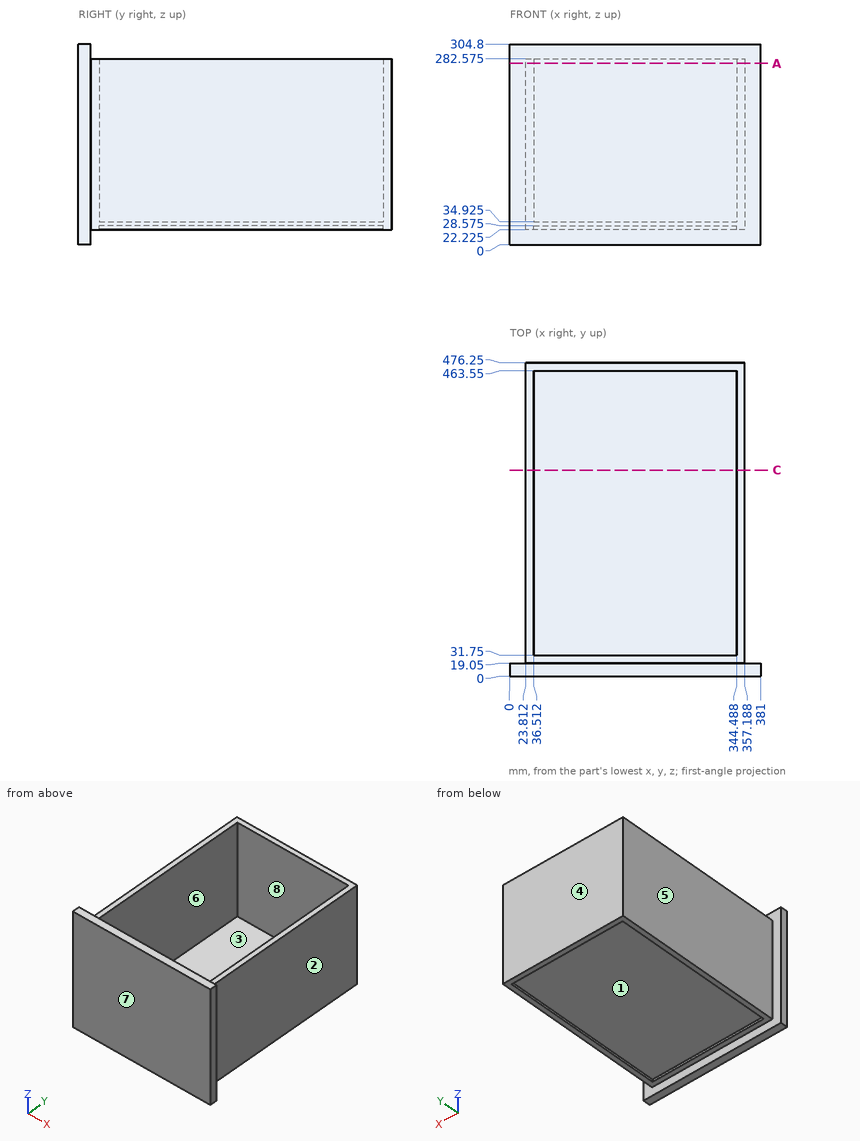
The figure shows three views and two pictorial views of one solid part (mm, origin at its lowest corner). Answer the questions. A direction names the side the tool comes from. Round coordinates to 2 decimals unless told otherwise and drop trailing zeros. Write each loop counter-clockwise with the first axis right and the second up, starting at its lowest first coordinate (ties: lowest second). Pieces come first, ordered by that corner, then holes. Notation, with made-up numbers: (38.5, 78) - (61.5, 78) arc R24 ccw to (61.5, 112) - close; hole circle Ø11 at (-38.75, 21). An arc over 180 degrees is marked (long way). Answer in a Markdown table with one row per item. Add a question column.
1. Find the intervals of material crossed by line 1 along X through (y, z) = (66, 204); line 2 along Y through (x, z) = (177.5, 228); line 3 along Z through (x, y) = (215.5, 319) (1 decimal), in increasing order. Write a range as from..to.
2. The mould has two halves that part along X. Classify the marked faces 5, 6, 7 and 8: +X half, -X half, draft (parallel to the pull), parting line (faces both ways), or undercut.
3. A cutting plane is placed at C-C, the plane y = 313. Determine the outline of the cut face in (x, z) (1 decimal), and give its area (3 significant figures).
4. Given pin 1 (1.9 mm diameter, centred on y = 310, z = 24.5, fed in from +X); pin 2 (5 mm diameter, centred on x = 236.5, y = 385, fed in from +Z) (1 decimal); pin 3 (7 mm diameter, centred on y = 245, z = 26, fed in from -X), each flat-ended and moving along its own axis, determine where each tip first touches the part or whether it passes through.
5. For the marked faces 1, 2, 3 and 4, determine the directions among +Z, -Z, +X, -X, +Y, -Y from which every point of the face is accessible in a straight line to the end or side of a thin tool.
6. A cutting plane is placed at A-A, the plane z = 275.5. Determine the outline of the cut face in (x, y), and give its area (3 significant figures).
Worked out:
| question | item | result |
|---|---|---|
| 1 | line 1 | 23.81..36.51, 344.49..357.19 |
| 1 | line 2 | 0..31.75, 463.55..476.25 |
| 1 | line 3 | 28.6..34.9 |
| 2 | face 5 | -X half |
| 2 | face 6 | undercut |
| 2 | face 7 | draft |
| 2 | face 8 | undercut |
| 3 | outline | (23.8, 22.2) - (36.5, 22.2) - (36.5, 28.6) - (344.5, 28.6) - (344.5, 22.2) - (357.2, 22.2) - (357.2, 282.6) - (344.5, 282.6) - (344.5, 34.9) - (36.5, 34.9) - (36.5, 282.6) - (23.8, 282.6) - close |
| 3 | area | 8,570 mm^2 |
| 4 | pin 1 | x = 357.19 |
| 4 | pin 2 | z = 34.9 |
| 4 | pin 3 | x = 23.81 |
| 5 | face 1 | -Z |
| 5 | face 2 | +Z, -Z, +X, +Y |
| 5 | face 3 | +Z |
| 5 | face 4 | +Z, -Z, +X, -X, +Y |
| 6 | outline | (0, 0) - (381, 0) - (381, 19.05) - (357.19, 19.05) - (357.19, 476.25) - (23.81, 476.25) - (23.81, 19.05) - (0, 19.05) - close; hole (36.51, 31.75) - (344.49, 31.75) - (344.49, 463.55) - (36.51, 463.55) - close |
| 6 | area | 26,700 mm^2 |
